The listing builds one solid part. Answer for the finished solid, in the listing's coordinates (mm). Face numbers are marked on the shaded views. Give positions to 0.01 mm unless a question says otherwise; leave off trailing zeros. Write each loop counter-clockwise with the first axis right and the second up, starting at its lowest first coordinate (ties: lowest second). Pieces come first, ordered by that corner, then holes.
```python
from build123d import *

# Parameters (mm, degrees)
F0_R      = 25.4
F1_DEPTH  = 177.8
F2_R      = 7.9375
F3_DEPTH  = 240.792
F4_R      = 22.225
F4_R_2    = 11.1125
F5_DEPTH  = 171.45
F6_R      = 28.604264
F6_R_2    = 14.624006
F7_DEPTH  = 3.175
F8_R      = 4.7625
F9_DEPTH  = 34.544
F10_R     = 11.060578
F10_R_2   = 8.077609
F11_DEPTH = 130.556


with BuildPart() as f1:
    # F0 (on Top) → F1 (new body)
    with BuildSketch(Plane.XY):
        Circle(F0_R)
    extrude(amount=F1_DEPTH)

    # F2 (on face) → F3 (cut)
    with BuildSketch(Plane.XY.offset(177.8)):
        Circle(F2_R)
    extrude(amount=-F3_DEPTH, mode=Mode.SUBTRACT)

    # F4 (on face) → F5 (cut)
    with BuildSketch(Plane.XY.offset(177.8)):
        Circle(F4_R)
        Circle(F4_R_2, mode=Mode.SUBTRACT)
    extrude(amount=-F5_DEPTH, mode=Mode.SUBTRACT)

    # F6 (on face) → F7 (cut)
    with BuildSketch(Plane.XY.offset(177.8)):
        Circle(F6_R)
        Circle(F6_R_2, mode=Mode.SUBTRACT)
    extrude(amount=-F7_DEPTH, mode=Mode.SUBTRACT)

    # F8 (on Front) → F9 (cut)
    with BuildSketch(Plane.XZ):
        with Locations((0, 57.984043)):
            Circle(F8_R)
    extrude(amount=F9_DEPTH, mode=Mode.SUBTRACT)

    # F10 (on face) → F11 (join)
    with BuildSketch(Plane.XY.offset(177.8)):
        Circle(F10_R)
        Circle(F10_R_2, mode=Mode.SUBTRACT)
    extrude(amount=-F11_DEPTH)


solid = f1.part
```
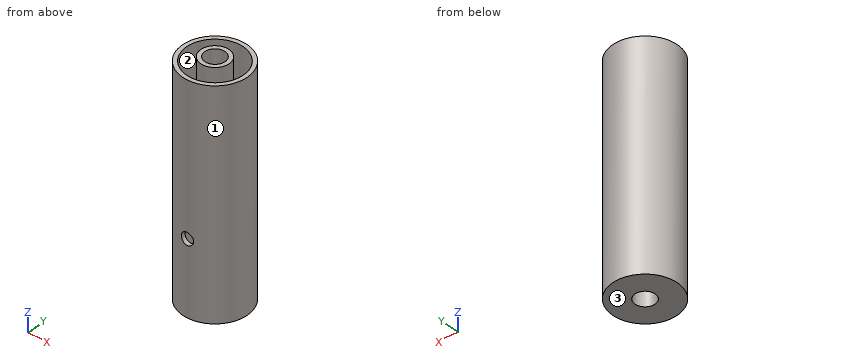
Item 1: Determine the mould class of the marked faces 1, 2 and 3 for opening direction Y: pulls with the +Y half, pulls with the -Y half, needs draft (parallel to the pull), parting line crosses it, or undercut.
Conclusion:
face 1: parting line crosses it
face 2: undercut
face 3: needs draft
Item 2: A cutting plane is placed at B-B, the plane x = 0. Count the separate pieces of the cut face and the enclosed holes in it, plus the area to 3 significant figures.
Conclusion:
separate pieces: 3
enclosed holes: 0
area: 2,350 mm2
Item 3: Consider probe 1 along Y at (x, z) = (0, 117) (1 decimal); probe 2 along Y at (x, z) = (-6, 52); probe 3 along X at (y, z) = (9.5, 133). Determine where each line is inside the solid, lowest interval first.
Conclusion:
probe 1: y = -25.4 to -22.2, -11.1 to -7.9, 7.9 to 11.1, 22.2 to 25.4
probe 2: y = -24.68 to -21.4, -9.35 to -5.2, 5.2 to 9.35, 21.4 to 24.68
probe 3: x = -23.56 to -20.09, -5.77 to 5.77, 20.09 to 23.56
Item 4: A cutting plane is placed at D-D, the plane y = 15.5. Give the vertices of the cut face in (x, z) (3 decimals), plus the area to 3 significant figures.
Conclusion:
outline: (-20.122, 0) - (20.122, 0) - (20.122, 174.625) - (15.928, 174.625) - (15.928, 6.35) - (-15.928, 6.35) - (-15.928, 174.625) - (-20.122, 174.625) - close
area: 1,670 mm2
Item 5: Each of these flat-tipped pins is pushed along its axis until it touches: P1, Ø6, axis at y = -12.5, z = 155.5, coming from the -X side; P2, Ø8.5, axis at x = 0, z = 57.98, coming from the -Y side; P3, Ø4, axis at x = 0.5, z = 45.5, coming from the +Y side. Where does it stop, or does it pass through?
Conclusion:
P1: stops at x = -23.56
P2: stops at y = -11.06
P3: stops at y = 25.4
